Check sheet for the modelled part. Datum: model origin and axes. Units: mm. Face numbers are marked on the shaded views. A direction names the side the tool comes from. Give positions to 0.01 mm unless a question says otherwise; leave off trailing zeros. Loops run counter-clockwise (first coordinate to the right, second up) from the corner with the lowest first, then second, coordinate; pieces in that order, holes last. Notation, with made-up numbers: (51, 76.5) - (92, 76.5) arc R12 cw to (92, 84.5) - close; hole circle Ø3 at (17, 23). An arc over 180 degrees is marked (long way). Use one line per item in the form item = value.
from build123d import *

# Parameters (mm, degrees)
BOX008_W         = 2
BOX008_H         = 3.3
BOX008_DEPTH     = 6
EXTRUDE004_DEPTH = 4.8


with BuildPart() as box008:
    # Box008 → Box008 (new body)
    with BuildSketch(Plane(origin=(1, 0, -0.5), x_dir=(1, 0, 0), z_dir=(0, 0, 1))):
        with Locations((1, 1.65)):
            Rectangle(BOX008_W, BOX008_H)
    extrude(amount=BOX008_DEPTH)


with BuildPart() as obj1:
    # Sketch002 → Extrude004 (new body)
    with BuildSketch(Plane.XZ):
        Polygon((2.309699, 1.35299), (2.309699, 3.266407), (0.956709, 4.619398), (-0.956709, 4.619398), (-2.309699, 3.266407), (-2.309699, 1.35299), (-0.956709, 0), (0.956709, 0), align=None)
    extrude(amount=-EXTRUDE004_DEPTH)

    # Cut: cut Box008
    add(box008.part, mode=Mode.SUBTRACT)


solid = obj1.part
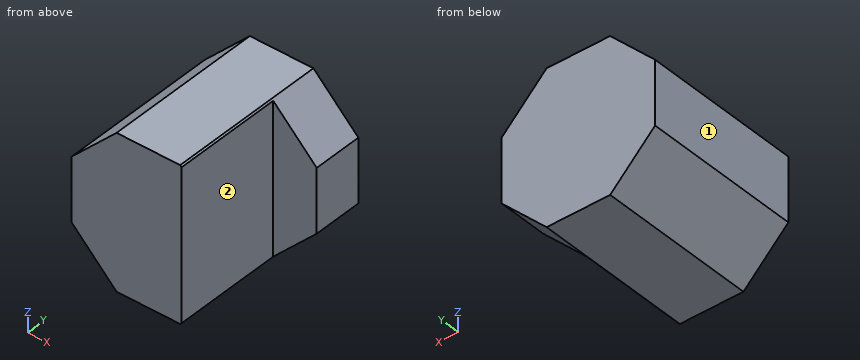
Item 1: Gauge pin test, flat end, axial feed: P1, Ø1.6, axis at y = 1.5, z = 2.5, coming from the +X side. Record the tip position at first contact, or that the pin passes through.
Answer block:
P1 = 1
Item 2: Section check D-D on y = 2.25. Record the boundary of the cut face in (x, z).
Answer block:
outline = (-2.31, 1.35) - (-0.96, 0) - (0.96, 0) - (1, 0.04) - (1, 4.58) - (0.96, 4.62) - (-0.96, 4.62) - (-2.31, 3.27) - close
Item 3: Section check A-A on y = 4.55. Record the boundary of the cut face in (x, z).
Answer block:
outline = (-2.31, 1.35) - (-0.96, 0) - (0.96, 0) - (2.31, 1.35) - (2.31, 3.27) - (0.96, 4.62) - (-0.96, 4.62) - (-2.31, 3.27) - close
Item 4: Section check C-C on x = -1.7. Record the boundary of the cut face in (y, z).
Answer block:
outline = (0, 0.74) - (4.8, 0.74) - (4.8, 3.88) - (0, 3.88) - close
Item 5: Thickness scan on L1, parallel to Z at x = -1, y = 2.45; L2, parallel to X at y = 0.75, z = 3.05; L3, parallel to Y at x = 1.5, z = 3.7. Record the ranges inside material, lowest first.
Answer block:
L1 = 0.04 to 4.58
L2 = -2.31 to 1
L3 = 3.3 to 4.8
Item 6: Access from +Z, -Z, +X, -X, +Y, -Y to the whole of each face (thin tool, end or side, straight path). Record for the marked faces 1 and 2.
Answer block:
face_1 = +Z, -Z, -X, +Y, -Y
face_2 = +Z, -Z, +X, -Y
Item 7: Section check B-B on z = 2.35. Record the boundary of the cut face in (x, y).
Answer block:
outline = (-2.31, 0) - (1, 0) - (1, 3.3) - (2.31, 3.3) - (2.31, 4.8) - (-2.31, 4.8) - close
